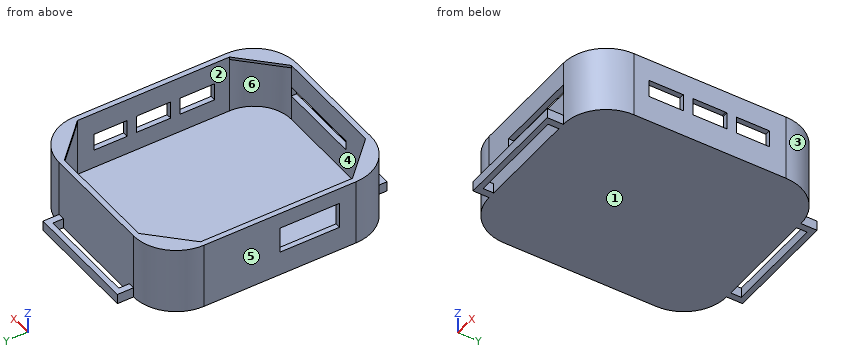
from build123d import *

# Parameters (mm, degrees)
EXTRUDE_2_DEPTH      = 1.5
EXTRUDE_4_DEPTH      = 11
EXTRUDE_START        = -0.5
EXTRUDE_7_DEPTH      = 0.5
EXTRUDE_8_DEPTH      = 0.5
EXTRUDE_9_DEPTH      = 0.5
SKETCH_12_W          = 4.897675457
SKETCH_12_H          = 11.127806736
CUT_EXTRUDE_3_DEPTH  = 3
SKETCH_13_W          = 3.241108758
SKETCH_13_H          = 6.19411896
CUT_EXTRUDE_4_DEPTH  = 3
SKETCH_14_W          = 3.313133397
SKETCH_14_H          = 6.122094321
CUT_EXTRUDE_5_DEPTH  = 3
SKETCH_15_W          = 2.880985563
SKETCH_15_H          = 6.266143599
CUT_EXTRUDE_6_DEPTH  = 3
SKETCH_16_W          = 15.721601541
SKETCH_16_H          = 1.836163931
CUT_EXTRUDE_7_DEPTH  = 3
SKETCH_19_W          = 3.275209086
SKETCH_19_H          = 6.371405254
SKETCH_19_H_2        = 6.414210644
CUT_EXTRUDE_10_DEPTH = 3
EXTRUDE_10_DEPTH     = 0.5
SKETCH_21_W          = 21.34
SKETCH_21_H          = 1.867544815
EXTRUDE_11_DEPTH     = 3
SKETCH_22_W          = 18.717201221
SKETCH_22_H          = 1.991492088
CUT_EXTRUDE_12_DEPTH = 3
SKETCH_23_W          = 21.381625352
SKETCH_23_H          = 3
EXTRUDE_12_DEPTH     = 1.87
SKETCH_24_W          = 18.956438282
SKETCH_24_H          = 1.976854412
CUT_EXTRUDE_13_DEPTH = 1.87


with BuildPart() as part:
    # 草图1 → 凸台-拉伸2 (new body)
    with BuildSketch(Plane.XY):
        with BuildLine():
            Line((-10.67, 22.215), (10.67, 22.215))
            ThreePointArc((10.67, 22.215), (16.326854249, 19.871854249), (18.67, 14.215))
            Line((18.67, 14.215), (18.67, -14.215))
            ThreePointArc((18.67, -14.215), (16.326854249, -19.871854249), (10.67, -22.215))
            Line((10.67, -22.215), (-10.67, -22.215))
            ThreePointArc((-10.67, -22.215), (-16.326854249, -19.871854249), (-18.67, -14.215))
            Line((-18.67, -14.215), (-18.67, 14.215))
            ThreePointArc((-18.67, 14.215), (-16.326854249, 19.871854249), (-10.67, 22.215))
        make_face()
    extrude(amount=EXTRUDE_2_DEPTH)

    # 草图4 → 凸台-拉伸4 (add)
    with BuildSketch(Plane.XY.offset(1.5)):
        with BuildLine():
            Line((18.67, -14.215), (18.67, 14.215))
            ThreePointArc((18.67, 14.215), (16.326854249, 19.871854249), (10.67, 22.215))
            Line((10.67, 22.215), (-10.67, 22.215))
            ThreePointArc((-10.67, 22.215), (-16.326854249, 19.871854249), (-18.67, 14.215))
            Line((-18.67, 14.215), (-18.67, -14.215))
            ThreePointArc((-18.67, -14.215), (-16.326854249, -19.871854249), (-10.67, -22.215))
            Line((-10.67, -22.215), (10.67, -22.215))
            ThreePointArc((10.67, -22.215), (16.326854249, -19.871854249), (18.67, -14.215))
        make_face()
        with BuildLine():
            Line((17.67, -14.215), (17.67, 14.215))
            ThreePointArc((17.67, 14.215), (15.619747468, 19.164747468), (10.67, 21.215))
            Line((10.67, 21.215), (-10.67, 21.215))
            ThreePointArc((-10.67, 21.215), (-15.619747468, 19.164747468), (-17.67, 14.215))
            Line((-17.67, 14.215), (-17.67, -14.215))
            ThreePointArc((-17.67, -14.215), (-15.619747468, -19.164747468), (-10.67, -21.215))
            Line((-10.67, -21.215), (10.67, -21.215))
            ThreePointArc((10.67, -21.215), (15.619747468, -19.164747468), (17.67, -14.215))
        make_face(mode=Mode.SUBTRACT)
    extrude(amount=EXTRUDE_4_DEPTH)

    # 草图8 → 凸台-拉伸7 (add)
    with BuildSketch(Plane.XY.offset(12.5).offset(EXTRUDE_START)):
        with BuildLine():
            Line((-17.67, -14.215), (-10.67, -21.215))
            ThreePointArc((-10.67, -21.215), (-15.619747468, -19.164747468), (-17.67, -14.215))
        make_face()
    extrude(amount=EXTRUDE_7_DEPTH)

    # 草图9 → 凸台-拉伸8 (add)
    with BuildSketch(Plane.XY.offset(12.5).offset(EXTRUDE_START)):
        with BuildLine():
            Line((10.67, 21.215), (17.67, 14.215))
            ThreePointArc((17.67, 14.215), (15.619747468, 19.164747468), (10.67, 21.215))
        make_face()
    extrude(amount=EXTRUDE_8_DEPTH)

    # 草图10 → 凸台-拉伸9 (add)
    with BuildSketch(Plane.XY.offset(12.5).offset(EXTRUDE_START)):
        with BuildLine():
            Line((17.67, -14.215), (10.67, -21.215))
            ThreePointArc((10.67, -21.215), (15.619747468, -19.164747468), (17.67, -14.215))
        make_face()
    extrude(amount=EXTRUDE_9_DEPTH)

    # 草图12 → 切除-拉伸3 (cut)
    with BuildSketch(Plane.ZY.offset(18.67)):
        with Locations((7.050780577, -5.563903368)):
            Rectangle(SKETCH_12_W, SKETCH_12_H)
    extrude(amount=-CUT_EXTRUDE_3_DEPTH, mode=Mode.SUBTRACT)

    # 草图13 → 切除-拉伸4 (cut)
    with BuildSketch(Plane(origin=(18.67, 0, 0), x_dir=(0, 0, -1), z_dir=(1, 0, 0))):
        with Locations((-6.646601976, 8.030747256)):
            Rectangle(SKETCH_13_W, SKETCH_13_H)
    extrude(amount=-CUT_EXTRUDE_4_DEPTH, mode=Mode.SUBTRACT)

    # 草图14 → 切除-拉伸5 (cut)
    with BuildSketch(Plane(origin=(18.67, 0, 0), x_dir=(0, 0, -1), z_dir=(1, 0, 0))):
        with Locations((-6.690937152, -0.144049279)):
            Rectangle(SKETCH_14_W, SKETCH_14_H)
    extrude(amount=-CUT_EXTRUDE_5_DEPTH, mode=Mode.SUBTRACT)

    # 草图15 → 切除-拉伸6 (cut)
    with BuildSketch(Plane(origin=(18.67, 0, 0), x_dir=(0, 0, -1), z_dir=(1, 0, 0))):
        with Locations((-6.664861945, -8.210808854)):
            Rectangle(SKETCH_15_W, SKETCH_15_H)
    extrude(amount=-CUT_EXTRUDE_6_DEPTH, mode=Mode.SUBTRACT)

    # 草图16 → 切除-拉伸7 (cut)
    with BuildSketch(Plane.XZ.offset(22.215)):
        with Locations((2.809199229, 7.168081965)):
            Rectangle(SKETCH_16_W, SKETCH_16_H)
    extrude(amount=-CUT_EXTRUDE_7_DEPTH, mode=Mode.SUBTRACT)

    # 草图19 → 切除-拉伸10 (cut)
    with BuildSketch(Plane(origin=(18.67, 0, 0), x_dir=(0, 0, -1), z_dir=(1, 0, 0))):
        with Locations((-6.671974996, -0.019393812)):
            Rectangle(SKETCH_19_W, SKETCH_19_H)
        with Locations((-6.671974996, -8.200049753)):
            Rectangle(SKETCH_19_W, SKETCH_19_H_2)
    extrude(amount=-CUT_EXTRUDE_10_DEPTH, mode=Mode.SUBTRACT)

    # 草图20 → 凸台-拉伸10 (add)
    with BuildSketch(Plane.XY.offset(12.5).offset(EXTRUDE_START)):
        with BuildLine():
            Line((-10.67, 21.215), (-17.67, 14.215))
            ThreePointArc((-17.67, 14.215), (-15.619747468, 19.164747468), (-10.67, 21.215))
        make_face()
    extrude(amount=EXTRUDE_10_DEPTH)

    # 草图21 → 凸台-拉伸11 (add)
    with BuildSketch(Plane(origin=(0, -22.215, 0), x_dir=(-1, 0, 0), z_dir=(0, -1, 0))):
        with Locations((0, -0.933772408)):
            Rectangle(SKETCH_21_W, SKETCH_21_H)
    extrude(amount=EXTRUDE_11_DEPTH)

    # 草图22 → 切除-拉伸12 (cut)
    with BuildSketch(Plane.XY.offset(1.867544815)):
        with Locations((0.035890498, -23.210746044)):
            Rectangle(SKETCH_22_W, SKETCH_22_H)
    extrude(amount=-CUT_EXTRUDE_12_DEPTH, mode=Mode.SUBTRACT)

    # 草图23 → 凸台-拉伸12 (add)
    with BuildSketch(Plane(origin=(-10.67, -22.215, 0), x_dir=(-1, 0, 0), z_dir=(0, 0, -1))):
        with Locations((-10.649187324, 45.93)):
            Rectangle(SKETCH_23_W, SKETCH_23_H)
    extrude(amount=-EXTRUDE_12_DEPTH)

    # 草图24 → 切除-拉伸13 (cut)
    with BuildSketch(Plane.XY.offset(1.87)):
        with Locations((-0.045973823, 23.203427206)):
            Rectangle(SKETCH_24_W, SKETCH_24_H)
    extrude(amount=-CUT_EXTRUDE_13_DEPTH, mode=Mode.SUBTRACT)


solid = part.part
For this review, take the finished solid that the model builds, in its own axes (mm). Face numbers are marked on the shaded views. A direction names the side the tool comes from. Give positions to 0.01 mm unless a question says otherwise; leave off trailing zeros. Order: outer loops, then holes, each group sorted by start corner. A loop starts at its lowest first (then second) coordinate and runs counter-clockwise, first axis right, second up. Notation, with made-up numbers: (4, 79) - (41, 79) arc R18 ccw to (41, 91) - close; hole circle Ø6 at (34.25, 33.5). An arc over 180 degrees is marked (long way). Answer as a JSON object with one key per item and string values. Group by question number.
Item 1: Draft analysis for pull direction X (two halves, no side actions). For the marked faces 1, 2 and 3, state which applies: pulls with the +X half, pulls with the -X half, needs draft (parallel to the pull), parting line crosses it, or undercut.
Item 2: Take a section at A-A on x = 5. Give the number of separate pieces and of enclosed holes in the cut face, and give its area (3 significant figures).
Item 3: Wall thickness on line 1 along Y through (x, z) = (-3, 2.25) (3 decimals); line 2 along X through (y, z) = (13, 3.5); line 3 along Z through (x, y) = (-10.5, -21): over which ranges is each line inside the solid? List them lowest first.
Item 4: Take a section at D-D on y = 4. Give the boundary of the cut face in (x, z), and give its area (3 significant figures).
Item 5: Take a section at C-C on z = 10.5. Give the boundary of the cut face in (x, y) (3 decimals).
Item 6: Machinability: for the marked faces 4, 5 and 6, which of the approach directions +Z, -Z, +X, -X, +Y, -Y give a long, thin tool a straight path to every point of the face, cutting with its end or side? Answer none if there is none.
Item 7: Clearance check with flat-ended pins moving along their axes: pin 1 Ø3.5 at (x, y) = (-2, -23) entering from +Z; pin 2 Ø3 at (x, y) = (7, -7.5) entering from +Z; pin 3 Ø6 at (x, z) = (2, 6) entering from +Y (3 decimals). State where each tip first meets the part, or that it passes through.
Reported:
{
 "1": {"face 1": "needs draft", "face 2": "undercut", "face 3": "pulls with the +X half"},
 "2": {"separate pieces": "4", "enclosed holes": "0", "area": "90.6 mm^2"},
 "3": {"line 1": "-22.215 to -21.215, 21.215 to 22.215", "line 2": "-18.67 to -17.67, 17.67 to 18.67", "line 3": "0 to 1.5"},
 "4": {"outline": "(-18.67, 0) - (18.67, 0) - (18.67, 12.5) - (17.67, 12.5) - (17.67, 1.5) - (-17.67, 1.5) - (-17.67, 12.5) - (-18.67, 12.5) - close", "area": "78.0 mm^2"},
 "5": {"outline": "(-18.67, -14.215) arc R8 ccw to (-10.67, -22.215) - (10.67, -22.215) arc R8 ccw to (18.67, -14.215) - (18.67, 14.215) arc R8 ccw to (10.67, 22.215) - (-10.67, 22.215) arc R8 ccw to (-18.67, 14.215) - close; hole (-17.67, -14.215) arc R7 ccw to (-10.67, -21.215) - (10.67, -21.215) arc R7 ccw to (17.67, -14.215) - (17.67, 14.215) arc R7 ccw to (10.67, 21.215) - (-10.67, 21.215) arc R7 ccw to (-17.67, 14.215) - close"},
 "6": {"face 4": "+Z", "face 5": "+Z, -Z, -X, +Y, -Y", "face 6": "none"},
 "7": {"pin 1": "z = 12.5", "pin 2": "z = 1.5", "pin 3": "y = 22.215"}
}
